Source: CAD feature listing. Evaluate the final solid. Frame: model axes, mm. Coordinates: 2 decimals unless noted, no trailing zeros. Write each loop counter-clockwise with the first axis right and the second up, starting at its lowest first coordinate (ties: lowest second). Pieces come first, ordered by that corner, then holes. Notation, with made-up numbers: (-31.75, 73) -> (-7.75, 73) arc R25 ccw to (-7.75, 103) -> close; hole circle Ø8 at (-13.75, 34). An arc over 180 degrees is marked (long way). One line per item, written item: value. Start each with the question number.
1. First-contact query: P1, Ø0.9, axis at x = 13.5, z = 1.5, coming from the -Y side; P2, Ø0.9, axis at y = 10.5, z = 2, coming from the -X side; P3, Ø0.9, axis at y = 1.5, z = 1, coming from the +X side. Flat tips, straight axial feed; report the tip coordinate or a pass-through.
2. Section query D-D, the plane x = -22. Output: boundary loops of the cut face in (y, z), and give its area (3 significant figures).
3. Section query C-C, the plane x = 23. Output: boundary loops of the cut face in (y, z).
4. Line query: line 1 (Y direction, x = 10, z = 1.75); line 2 (Y direction, x = -13, z = 1.7); line 3 (X direction, y = 14.5, z = 0.2). Output: solid intervals per line, ascending.
5. Section query B-B, the plane y = 24. Output: boundary loops of the cut face in (x, z), and give its area (3 significant figures).
6. Section query A-A, the plane z = 1.6. State how many separate pieces and enclosed holes the cut face has, and give its area (3 significant figures).
from build123d import *

# Parameters (mm, degrees)
ESQUISSE1_R                = 1.5
BOSS_EXTRU_1_DEPTH         = 3
ESQUISSE2_W                = 4
ESQUISSE2_H                = 3
ENL_V_MAT_EXTRU_2_DEPTH    = 3
R_P_TITION_LIN_AIRE1_COUNT = 5
R_P_TITION_LIN_AIRE1_PITCH = 8


with BuildPart() as part:
    # Esquisse1 → Boss.-Extru.1 (new body)
    with BuildSketch(Plane.XY):
        with BuildLine():
            Line((0, 17.5), (0, 0))
            Line((0, 0), (40, 0))
            ThreePointArc((40, 0), (28.284271247, 28.284271247), (0, 40))
            Line((0, 40), (-30, 40))
            Line((-30, 40), (-30, 17.5))
            Line((-30, 17.5), (0, 17.5))
        make_face()
        with Locations((10, 11)):
            Circle(ESQUISSE1_R, mode=Mode.SUBTRACT)
        with BuildLine():
            ThreePointArc((10, 22.5), (8.5, 24), (10, 25.5))
            ThreePointArc((10, 25.5), (20.253048327, 21.253048327), (24.5, 11))
            ThreePointArc((24.5, 11), (23, 9.5), (21.5, 11))
            ThreePointArc((21.5, 11), (18.131727984, 19.131727984), (10, 22.5))
        make_face(mode=Mode.SUBTRACT)
    extrude(amount=BOSS_EXTRU_1_DEPTH)

    # Esquisse2 → Enlèv. mat.-Extru.2 (cut)
    with BuildSketch(Plane.XY.offset(3)):
        with Locations((6, 1.5)):
            Rectangle(ESQUISSE2_W, ESQUISSE2_H)
    enl_v_mat_extru_2 = extrude(amount=-ENL_V_MAT_EXTRU_2_DEPTH, mode=Mode.SUBTRACT)

    # Répétition linéaire1: Enlèv. mat.-Extru.2 ×5
    with Locations(*[(i * R_P_TITION_LIN_AIRE1_PITCH, 0, 0) for i in range(1, R_P_TITION_LIN_AIRE1_COUNT)]):
        add(enl_v_mat_extru_2, mode=Mode.SUBTRACT)


solid = part.part
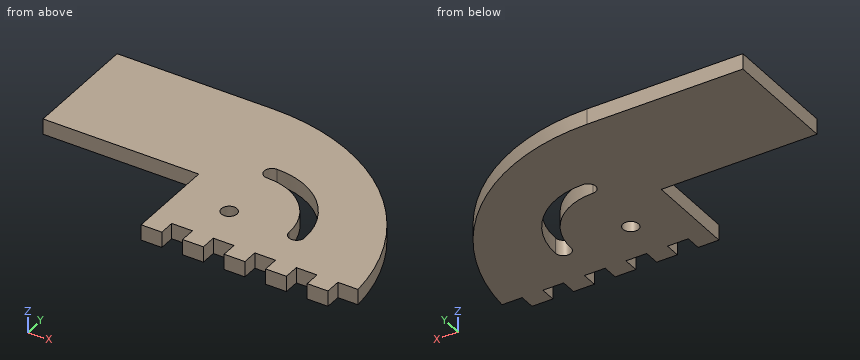
Computed values:
1. P1: stops at y = 3
1. P2: stops at x = 0
1. P3: stops at x = 36
2. outline: (17.5, 0) -> (40, 0) -> (40, 3) -> (17.5, 3) -> close
2. area: 67.5 mm²
3. outline: (3, 0) -> (9.5, 0) -> (9.5, 3) -> (3, 3) -> close; (17.42, 0) -> (32.73, 0) -> (32.73, 3) -> (17.42, 3) -> close
4. line 1: y = 0 to 9.5, 12.5 to 22.5, 25.5 to 38.73
4. line 2: y = 17.5 to 40
4. line 3: x = 0 to 20.95, 24.07 to 37.28
5. outline: (-30, 0) -> (8.5, 0) -> (8.5, 3) -> (-30, 3) -> close; (16.42, 0) -> (32, 0) -> (32, 3) -> (16.42, 3) -> close
5. area: 162 mm²
6. separate pieces: 1
6. enclosed holes: 2
6. area: 1,800 mm²
